Autodesk Inventor part; units mm, degrees
ref_plane "YZ Plane" through (0, 0, 0) normal (1, 0, 0) x (0, 1, 0)
ref_plane "XZ Plane" through (0, 0, 0) normal (0, 1, 0) x (-1, 0, 0)
ref_plane "XY Plane" through (0, 0, 0) normal (0, 0, 1) x (1, 0, 0)
sketch "Sketch1" plane through (0, 0, 0) normal (0, 1, 0) x (-1, 0, 0)
  line L0 (18, 16) -> (-18, 16)
  line L1 (-18, 16) -> (-18, -16)
  line L2 (-18, -16) -> (18, -16)
  line L3 (18, -16) -> (18, 16)
  line L4 (18, 16) -> (-18, -16) construction
  line L5 (-18, 16) -> (18, -16) construction
  point P0 (0, 0)
  dimension "d0" = 36
  dimension "d1" = 32
extrude "Extrusion1" add sketch "Sketch1" along normal blind 10
sketch "Sketch2" plane through (0, 0, 0) normal (0, -1, 0) x (1, 0, 0)
  circle A0 centre (6.95, 12.5) radius 1.2295
  circle A1 centre (6.95, -12.5) radius 1.2295
  circle A2 centre (-13.05, -12.5) radius 1.2295
  circle A3 centre (-13.05, 12.5) radius 1.2295
  line L0 (-24.1, 15) -> (18, 15)
  line L1 (-24.1, -15) -> (-24.1, 15)
  line L2 (18, -15) -> (-24.1, -15)
  line L3 (18, 15) -> (18, -15)
  point P0 (0, 0)
hole "Hole1" at (6.95, 0, -12.5) at (-13.05, 0, -12.5) at (6.95, 0, 12.5) at (-13.05, 0, 12.5) direction (0, 1, 0) diameter 3 end through all counterbore diameter 6 counterbore depth 3.5
sketch "Sketch3" plane through (0, 0, 0) normal (0, -1, 0) x (1, 0, 0)
  circle A0 centre (-13.05, 12.5) radius 3
  circle A1 centre (6.95, 12.5) radius 3
  circle A2 centre (-13.05, -12.5) radius 3
  circle A3 centre (6.95, -12.5) radius 3
  line L0 (18, 16) -> (18, -16)
  line L1 (-18, 16) -> (18, 16)
  line L2 (-18, -16) -> (-18, 16)
  line L3 (18, -16) -> (-18, -16)
  point P0 (0, 0)
  point P1 (5, 0)
  dimension "d11" = 5
hole "Hole2" at (5, 0, 0) direction (0, 1, 0) diameter 6.647 end through all
properties part number "LM Cart Braket" material "Aluminum 6061-AHC"
Design review of the part built by this model. Coordinates are the model's own, in mm. A direction names the side the tool comes from. Give positions to 0.01 mm unless a question says otherwise; leave off trailing zeros. Loops run counter-clockwise (first coordinate to the right, second up) from the corner with the lowest first, then second, coordinate; pieces in that order, holes last. Notation, with made-up numbers: M 60.5,33.5 L 97.5,33.5 A23 ccw 97.5,69.5 Z; hole C 58,35 d3. An arc over 180 degrees is marked long. Return JSON: item names as keys, results as strings. Group by question number.
Item 1: We need section B-B (x = -13.05). Give the boundary of the cut face in (y, z), and give its area (3 significant figures).
Item 2: For probe 1 along X at (y, z) = (0.7, -12.5); probe 2 along Z at (x, y) = (-13.05, 8); probe 3 along X at (y, z) = (7.5, -12.5), list the stretches that pass through material, from the lowest coordinate up.
Item 3: We need section C-C (z = 12.5). Give the boundary of the cut face in (x, y).
Item 4: We need section A-A (z = 0). Give the boundary of the cut face in (x, y).
Item 5: Tool access review of faces 1 (the cylindrical face through (-16.024, 1.774, -12.109)), 2 (the flat face through (18, 5, 0)): name each direction out of +Z, -Z, +X, -X, +Y, -Y from which nothing blocks a thin tool from reaching the whole face with its end or side.
Item 6: Mouldability with a two-part tool opening along X and no side actions: class faces 3 (the flat face through (0, 0, 0)), 4 (the cylindrical face through (8.775, 1.774, 14.881)), 5 (the flat face through (-18, 5, 0)) as released by +X, released by -X, zero draft, split by the parting line, or undercut.
Item 7: Insertion check: pin 1 Ø6 at (x, z) = (5, 0) entering from +Y; pin 2 Ø9.5 at (x, z) = (6.95, 12.5) entering from -Y; pin 3 Ø5.5 at (x, z) = (-13.05, -12.5) entering from -Y. Each pin has a flat end and moves straight along its axis. Give the tip position at first contact, or say it passes through.
Item 8: We need section D-D (y = 9). Give the boundary of the cut face in (x, z).
Output:
{
 "1": {"outline": "M 0,-16 L 10,-16 L 10,-14 L 3.5,-14 L 3.5,-15.5 L 0,-15.5 Z; M 0,-9.5 L 3.5,-9.5 L 3.5,-11 L 10,-11 L 10,11 L 3.5,11 L 3.5,9.5 L 0,9.5 Z; M 0,15.5 L 3.5,15.5 L 3.5,14 L 10,14 L 10,16 L 0,16 Z", "area": "239 mm^2"},
 "2": {"probe 1": "x = -18 to -16.05, -10.05 to 3.95, 9.95 to 18", "probe 2": "z = -16 to -14, -11 to 11, 14 to 16", "probe 3": "x = -18 to -14.55, -11.55 to 5.45, 8.45 to 18"},
 "3": {"outline": "M -18,0 L -16.05,0 L -16.05,3.5 L -14.55,3.5 L -14.55,10 L -18,10 Z; M -11.55,3.5 L -10.05,3.5 L -10.05,0 L 3.95,0 L 3.95,3.5 L 5.45,3.5 L 5.45,10 L -11.55,10 Z; M 8.45,3.5 L 9.95,3.5 L 9.95,0 L 18,0 L 18,10 L 8.45,10 Z"},
 "4": {"outline": "M -18,0 L 1.68,0 L 1.68,10 L -18,10 Z; M 8.32,0 L 18,0 L 18,10 L 8.32,10 Z"},
 "5": {"face 1": "-Y", "face 2": "+Z, -Z, +X, +Y, -Y"},
 "6": {"face 3": "zero draft", "face 4": "undercut", "face 5": "released by -X"},
 "7": {"pin 1": "passes through", "pin 2": "stops at y = 0", "pin 3": "stops at y = 3.5"},
 "8": {"outline": "M -18,-16 L 18,-16 L 18,16 L -18,16 Z; hole C -13.05,-12.5 d3; hole C -13.05,12.5 d3; hole C 5,0 d6.65; hole C 6.95,-12.5 d3; hole C 6.95,12.5 d3"}
}
